Source: CAD feature listing. Evaluate the final solid. Frame: model axes, mm. Give positions to 0.01 mm unless a question says otherwise; leave off trailing zeros. Order: outer loops, then holes, each group sorted by start corner. A loop starts at its lowest first (then second) coordinate and runs counter-clockwise, first axis right, second up.
```python
from build123d import *

# Parameters (mm, degrees)
SKETCH_F_R                   = 3.1
ESTRUSIONE_ESTRUSIONE1_DEPTH = 5


with BuildPart() as part:
    # Sketch f → Estrusione-Estrusione1 (new body)
    with BuildSketch(Plane.XY):
        with BuildLine():
            Line((0, 0), (0, 79))
            Line((0, 79), (179.5, 79))
            ThreePointArc((179.5, 79), (186.571067812, 76.071067812), (189.5, 69))
            Line((189.5, 69), (189.5, 58))
            ThreePointArc((189.5, 58), (190.671572875, 55.171572875), (193.5, 54))
            Line((193.5, 54), (255.5, 54))
            ThreePointArc((255.5, 54), (258.328427125, 55.171572875), (259.5, 58))
            Line((259.5, 58), (259.5, 69))
            ThreePointArc((259.5, 69), (262.428932188, 76.071067812), (269.5, 79))
            Line((269.5, 79), (449, 79))
            Line((449, 79), (449, 0))
            Line((449, 0), (0, 0))
        make_face()
        with Locations((11.5, 67.5)):
            Circle(SKETCH_F_R, mode=Mode.SUBTRACT)
        with Locations((437.5, 67.5)):
            Circle(SKETCH_F_R, mode=Mode.SUBTRACT)
        with Locations((11.5, 11.5)):
            Circle(SKETCH_F_R, mode=Mode.SUBTRACT)
        with Locations((437.5, 11.5)):
            Circle(SKETCH_F_R, mode=Mode.SUBTRACT)
    extrude(amount=ESTRUSIONE_ESTRUSIONE1_DEPTH)


solid = part.part
```
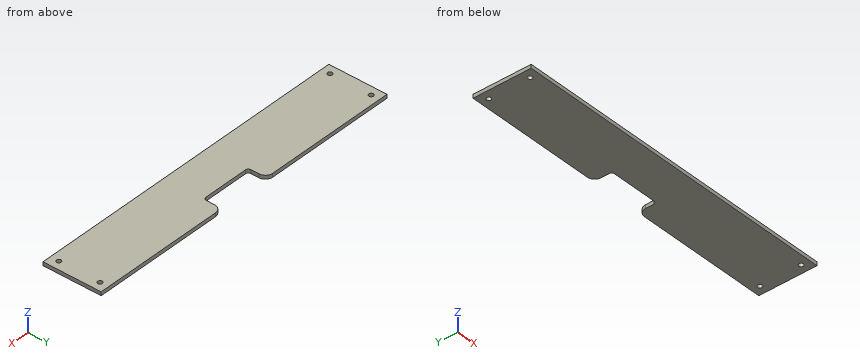
1) Material intervals for L1, parallel to Y at x = 11.5, z = 2.5; L2, parallel to X at y = 68.5, z = 0.8; L3, parallel to X at y = 58.5, z = 1, sorted ascending.
Report:
L1: y = 0 to 8.4, 14.6 to 64.4, 70.6 to 79
L2: x = 0 to 8.57, 14.43 to 189.5, 259.5 to 434.57, 440.43 to 449
L3: x = 0 to 189.5, 259.5 to 449
2) Section query A-A, the plane z = 2.25. Return the cut outline in (x, y).
Report:
outline: (0, 0) - (449, 0) - (449, 79) - (269.5, 79) arc R10 ccw to (259.5, 69) - (259.5, 58) arc R4 cw to (255.5, 54) - (193.5, 54) arc R4 cw to (189.5, 58) - (189.5, 69) arc R10 ccw to (179.5, 79) - (0, 79) - close; hole circle Ø6.2 at (11.5, 11.5); hole circle Ø6.2 at (11.5, 67.5); hole circle Ø6.2 at (437.5, 11.5); hole circle Ø6.2 at (437.5, 67.5)
3) Pin query (flat end, axial travel): pin 1 (5 mm diameter, centred on x = 437.5, y = 11.5, fed in from -Z); pin 2 (1.5 mm diameter, centred on x = 240, z = 4, fed in from +Y). Return the tip coordinate at first contact, or that it passes through.
Report:
pin 1: passes through
pin 2: stops at y = 54
